from build123d import *

# Parameters (mm, degrees)
SKETCH1_R           = 2.6035
BOSS_EXTRUDE1_DEPTH = 152.4


with BuildPart() as part:
    # Sketch1 → Boss-Extrude1 (new body)
    with BuildSketch(Plane.XY):
        with BuildLine():
            Line((-12.7, -12.7), (-4.343399971, -12.7))
            ThreePointArc((-4.343399971, -12.7), (-3.238499971, -11.5951), (-4.343399971, -10.4902))
            Line((-4.343399971, -10.4902), (-6.474794456, -10.4902))
            ThreePointArc((-6.474794456, -10.4902), (-7.413456061, -9.863006367), (-7.193214945, -8.75577951))
            Line((-7.193214945, -8.75577951), (-2.933235435, -4.4958))
            Line((-2.933235435, -4.4958), (2.933235435, -4.4958))
            Line((2.933235435, -4.4958), (7.193214945, -8.75577951))
            ThreePointArc((7.193214945, -8.75577951), (7.413456061, -9.863006367), (6.474794456, -10.4902))
            Line((6.474794456, -10.4902), (4.3434, -10.4902))
            ThreePointArc((4.3434, -10.4902), (3.2385, -11.5951), (4.3434, -12.7))
            Line((4.3434, -12.7), (12.7, -12.7))
            Line((12.7, -12.7), (12.7, -4.343399971))
            ThreePointArc((12.7, -4.343399971), (11.5951, -3.238499971), (10.4902, -4.343399971))
            Line((10.4902, -4.343399971), (10.4902, -6.474794456))
            ThreePointArc((10.4902, -6.474794456), (9.863006367, -7.413456061), (8.75577951, -7.193214945))
            Line((8.75577951, -7.193214945), (4.4958, -2.933235435))
            Line((4.4958, -2.933235435), (4.4958, 2.933235435))
            Line((4.4958, 2.933235435), (8.75577951, 7.193214945))
            ThreePointArc((8.75577951, 7.193214945), (9.863006367, 7.413456061), (10.4902, 6.474794456))
            Line((10.4902, 6.474794456), (10.4902, 4.3434))
            ThreePointArc((10.4902, 4.3434), (11.5951, 3.2385), (12.7, 4.3434))
            Line((12.7, 4.3434), (12.7, 12.7))
            Line((12.7, 12.7), (4.343399971, 12.7))
            ThreePointArc((4.343399971, 12.7), (3.238499971, 11.5951), (4.343399971, 10.4902))
            Line((4.343399971, 10.4902), (6.474794456, 10.4902))
            ThreePointArc((6.474794456, 10.4902), (7.413456061, 9.863006367), (7.193214945, 8.75577951))
            Line((7.193214945, 8.75577951), (2.933235435, 4.4958))
            Line((2.933235435, 4.4958), (-2.933235435, 4.4958))
            Line((-2.933235435, 4.4958), (-7.193214945, 8.75577951))
            ThreePointArc((-7.193214945, 8.75577951), (-7.413456061, 9.863006367), (-6.474794456, 10.4902))
            Line((-6.474794456, 10.4902), (-4.3434, 10.4902))
            ThreePointArc((-4.3434, 10.4902), (-3.2385, 11.5951), (-4.3434, 12.7))
            Line((-4.3434, 12.7), (-12.7, 12.7))
            Line((-12.7, 12.7), (-12.7, 4.343399971))
            ThreePointArc((-12.7, 4.343399971), (-11.5951, 3.238499971), (-10.4902, 4.343399971))
            Line((-10.4902, 4.343399971), (-10.4902, 6.474794456))
            ThreePointArc((-10.4902, 6.474794456), (-9.863006367, 7.413456061), (-8.75577951, 7.193214945))
            Line((-8.75577951, 7.193214945), (-4.4958, 2.933235435))
            Line((-4.4958, 2.933235435), (-4.4958, -2.933235435))
            Line((-4.4958, -2.933235435), (-8.75577951, -7.193214945))
            ThreePointArc((-8.75577951, -7.193214945), (-9.863006367, -7.413456061), (-10.4902, -6.474794456))
            Line((-10.4902, -6.474794456), (-10.4902, -4.3434))
            ThreePointArc((-10.4902, -4.3434), (-11.5951, -3.2385), (-12.7, -4.3434))
            Line((-12.7, -4.3434), (-12.7, -12.7))
        make_face()
        Circle(SKETCH1_R, mode=Mode.SUBTRACT)
    extrude(amount=-BOSS_EXTRUDE1_DEPTH)


solid = part.part
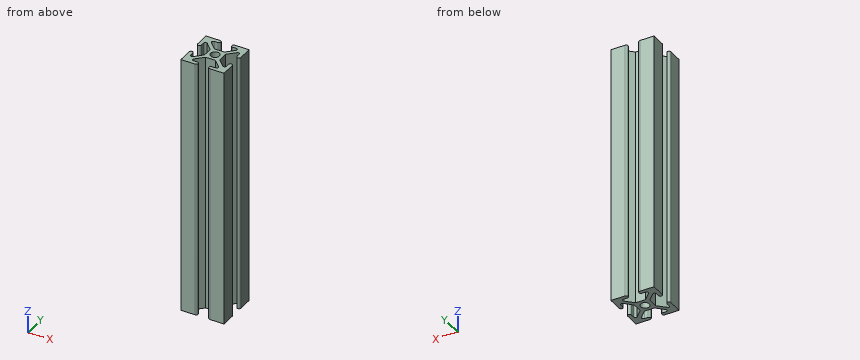
Can you work these out from the model? Positions are in its coordinate system, mm. Give positions to 0.01 mm unless a question says otherwise; leave off trailing zeros. Write each loop counter-clockwise with the first axis right and the second up, starting at its lowest first coordinate (ties: lowest second). Pieces come first, ordered by that corner, then holes. Notation, with made-up numbers: (1.5, 71.25) -> (60.5, 71.25) arc R28 ccw to (60.5, 110.25) -> close; hole circle Ø10 at (39, 19). An arc over 180 degrees is marked (long way). Answer as a JSON object with one key per item and string values. Group by question number.
Item 1: Please list where these lines run through material, in increasing order: line 1 (Y direction, x = 0, z = -60); line 2 (X direction, y = 3.5, z = -55); line 3 (Y direction, x = -5.5, z = -52.5). Write a range as [from, to].
Item 2: Suppose I cut it at A-A (x = 0). Please give me the cut outline in (y, z), plus the area to 3 significant figures.
Item 3: I'm going to push flat-ended pins straight in: P1, Ø8, axis at y = 4, z = -130, coming from the -X side; P2, Ø1.5, axis at x = 1, z = -120, coming from the +Y side; P3, Ø4.5, axis at y = -0.5, z = -51, coming from the +X side; P4, Ø4, axis at x = 1.5, z = -67, coming from the +Y side. Where does each tip first touch, or does it pass through?
Findings:
{
 "1": {"line 1": "y = [-4.5, -2.6], [2.6, 4.5]", "line 2": "x = [-12.31, -10.88], [-5.06, 5.06], [10.88, 12.31]", "line 3": "y = [-12.7, -10.49], [-7.06, -3.94], [3.94, 7.06], [10.49, 12.7]"},
 "2": {"outline": "(-4.5, -152.4) -> (-2.6, -152.4) -> (-2.6, 0) -> (-4.5, 0) -> close; (2.6, -152.4) -> (4.5, -152.4) -> (4.5, 0) -> (2.6, 0) -> close", "area": "577 mm²"},
 "3": {"P1": "stops at x = -12.7", "P2": "stops at y = 4.5", "P3": "stops at x = 4.5", "P4": "stops at y = 12.31"}
}
